Here's how the part is built. I have some questions about the finished solid (model axes, mm). Coordinates: 2 decimals unless noted, no trailing zeros. Write each loop counter-clockwise with the first axis right and the second up, starting at its lowest first coordinate (ties: lowest second). Pieces come first, ordered by that corner, then holes. Notation, with made-up numbers: M -28.5,75.25 L 0.5,75.25 A14 ccw 0.5,99.25 Z; hole C 74,44 d4. An arc over 180 degrees is marked long. Use one line per item in the form item = value. Start each with the question number.
1. Thinking about a two-plate mould opening in Y: for faces 1 (the face through (-2.17, -9.76, 0.49)), 2 (the face through (3.887, -1.591, -4.916)), which applies, released by +Y, released by -Y, zero draft, split by the parting line, or undercut?
2. Please list where these lines run through material, in increasing order: line 1 along Y through (x, z) = (0, -8); line 2 along X through (y, z) = (-6.75, -3); line 3 along Z through (x, y) = (3.5, -8.5). Write a range as [from, to].
3. I want a section at A-A, the plane x = 0. List the corners of the cut face in (y, z) for me.
4. I want a section at C-C, the plane x = 7.75. List the corners of the cut face in (y, z) for me.
5. I want a section at D-D, the plane z = 0.5. Count the separate pieces of the cut face and the enclosed holes in it, plus the area to 3 significant figures.
6. I'm going to push flat-ended pins straight in: pin 1 Ø0.5 at (x, z) = (-7.5, -4) entering from +Y; pin 2 Ø1.3 at (y, z) = (7, -2.5) entering from -X; pin 3 Ø0.5 at (x, z) = (2.5, -2.5) entering from +Y. Where does each tip first touch, or does it pass through?
from build123d import *

# Parameters (mm, degrees)
SKETCH1_R           = 10
BOSS_EXTRUDE1_DEPTH = 1
SKETCH2_R           = 9
BOSS_EXTRUDE2_DEPTH = 11
SKETCH3_R           = 1
CUT_EXTRUDE2_DEPTH  = 19.547236991


with BuildPart() as part:
    # Sketch1 → Boss-Extrude1 (new body)
    with BuildSketch(Plane.XY):
        Circle(SKETCH1_R)
    extrude(amount=BOSS_EXTRUDE1_DEPTH)

    # Sketch2 → Boss-Extrude2 (add)
    with BuildSketch(Plane(origin=(0, 0, 0), x_dir=(-1, 0, 0), z_dir=(0, 0, -1))):
        Circle(SKETCH2_R)
    extrude(amount=BOSS_EXTRUDE2_DEPTH)

    # Sketch3 → Cut-Extrude2 (cut, through all)
    with BuildSketch(Plane.XY.offset(1)):
        Circle(SKETCH3_R)
        with BuildLine():
            ThreePointArc((-1.754992877, 0.4), (-1.272792206, 1.272792206), (-0.4, 1.754992877))
            Line((-0.4, 1.754992877), (-0.4, 3.376388603))
            ThreePointArc((-0.4, 3.376388603), (-2.404163056, 2.404163056), (-3.376388603, 0.4))
            Line((-3.376388603, 0.4), (-1.754992877, 0.4))
        make_face()
        with BuildLine():
            Line((0.4, 3.376388603), (0.4, 1.754992877))
            ThreePointArc((0.4, 1.754992877), (1.272792206, 1.272792206), (1.754992877, 0.4))
            Line((1.754992877, 0.4), (3.376388603, 0.4))
            ThreePointArc((3.376388603, 0.4), (2.404163056, 2.404163056), (0.4, 3.376388603))
        make_face()
        with BuildLine():
            Line((3.376388603, -0.4), (1.754992877, -0.4))
            ThreePointArc((1.754992877, -0.4), (1.272792206, -1.272792206), (0.4, -1.754992877))
            Line((0.4, -1.754992877), (0.4, -3.376388603))
            ThreePointArc((0.4, -3.376388603), (2.404163056, -2.404163056), (3.376388603, -0.4))
        make_face()
        with BuildLine():
            ThreePointArc((-0.4, -1.754992877), (-1.272792206, -1.272792206), (-1.754992877, -0.4))
            Line((-1.754992877, -0.4), (-3.376388603, -0.4))
            ThreePointArc((-3.376388603, -0.4), (-2.404163056, -2.404163056), (-0.4, -3.376388603))
            Line((-0.4, -3.376388603), (-0.4, -1.754992877))
        make_face()
        with BuildLine():
            ThreePointArc((0.4, 4.180908992), (1.607270416, 3.880294037), (2.673506387, 3.239191812))
            Line((2.673506387, 3.239191812), (3.808611797, 4.374297222))
            ThreePointArc((3.808611797, 4.374297222), (2.219563908, 5.358501289), (0.4, 5.786190457))
            Line((0.4, 5.786190457), (0.4, 4.180908992))
        make_face()
        with BuildLine():
            ThreePointArc((-2.673506387, 3.239191812), (-1.607270416, 3.880294037), (-0.4, 4.180908992))
            Line((-0.4, 4.180908992), (-0.4, 5.786190457))
            ThreePointArc((-0.4, 5.786190457), (-2.219563908, 5.358501289), (-3.808611797, 4.374297222))
            Line((-3.808611797, 4.374297222), (-2.673506387, 3.239191812))
        make_face()
        with BuildLine():
            ThreePointArc((-4.180908992, 0.4), (-3.880294037, 1.607270416), (-3.239191812, 2.673506387))
            Line((-3.239191812, 2.673506387), (-4.374297222, 3.808611797))
            ThreePointArc((-4.374297222, 3.808611797), (-5.358501289, 2.219563908), (-5.786190457, 0.4))
            Line((-5.786190457, 0.4), (-4.180908992, 0.4))
        make_face()
        with BuildLine():
            ThreePointArc((-3.239191812, -2.673506387), (-3.880294037, -1.607270416), (-4.180908992, -0.4))
            Line((-4.180908992, -0.4), (-5.786190457, -0.4))
            ThreePointArc((-5.786190457, -0.4), (-5.358501289, -2.219563908), (-4.374297222, -3.808611797))
            Line((-4.374297222, -3.808611797), (-3.239191812, -2.673506387))
        make_face()
        with BuildLine():
            Line((-0.4, -5.786190457), (-0.4, -4.180908992))
            ThreePointArc((-0.4, -4.180908992), (-1.607270416, -3.880294037), (-2.673506387, -3.239191812))
            Line((-2.673506387, -3.239191812), (-3.808611797, -4.374297222))
            ThreePointArc((-3.808611797, -4.374297222), (-2.219563908, -5.358501289), (-0.4, -5.786190457))
        make_face()
        with BuildLine():
            Line((3.808611797, -4.374297222), (2.673506387, -3.239191812))
            ThreePointArc((2.673506387, -3.239191812), (1.607270416, -3.880294037), (0.4, -4.180908992))
            Line((0.4, -4.180908992), (0.4, -5.786190457))
            ThreePointArc((0.4, -5.786190457), (2.219563908, -5.358501289), (3.808611797, -4.374297222))
        make_face()
        with BuildLine():
            Line((5.786190457, -0.4), (4.180908992, -0.4))
            ThreePointArc((4.180908992, -0.4), (3.880294037, -1.607270416), (3.239191812, -2.673506387))
            Line((3.239191812, -2.673506387), (4.374297222, -3.808611797))
            ThreePointArc((4.374297222, -3.808611797), (5.358501289, -2.219563908), (5.786190457, -0.4))
        make_face()
        with BuildLine():
            Line((4.374297222, 3.808611797), (3.239191812, 2.673506387))
            ThreePointArc((3.239191812, 2.673506387), (3.880294037, 1.607270416), (4.180908992, 0.4))
            Line((4.180908992, 0.4), (5.786190457, 0.4))
            ThreePointArc((5.786190457, 0.4), (5.358501289, 2.219563908), (4.374297222, 3.808611797))
        make_face()
        with BuildLine():
            ThreePointArc((8.190238092, 0.4), (7.575812167, 3.138004145), (6.074215607, 5.508530182))
            Line((6.074215607, 5.508530182), (4.941168592, 4.375483167))
            ThreePointArc((4.941168592, 4.375483167), (6.097604915, 2.525710654), (6.587867637, 0.4))
            Line((6.587867637, 0.4), (8.190238092, 0.4))
        make_face()
        with BuildLine():
            ThreePointArc((5.508530182, 6.074215607), (3.138004145, 7.575812167), (0.4, 8.190238092))
            Line((0.4, 8.190238092), (0.4, 6.587867637))
            ThreePointArc((0.4, 6.587867637), (2.525710654, 6.097604915), (4.375483167, 4.941168592))
            Line((4.375483167, 4.941168592), (5.508530182, 6.074215607))
        make_face()
        with BuildLine():
            Line((-0.4, 6.587867637), (-0.4, 8.190238092))
            ThreePointArc((-0.4, 8.190238092), (-3.138004145, 7.575812167), (-5.508530182, 6.074215607))
            Line((-5.508530182, 6.074215607), (-4.375483167, 4.941168592))
            ThreePointArc((-4.375483167, 4.941168592), (-2.525710654, 6.097604915), (-0.4, 6.587867637))
        make_face()
        with BuildLine():
            Line((-4.941168592, 4.375483167), (-6.074215607, 5.508530182))
            ThreePointArc((-6.074215607, 5.508530182), (-7.575812167, 3.138004145), (-8.190238092, 0.4))
            Line((-8.190238092, 0.4), (-6.587867637, 0.4))
            ThreePointArc((-6.587867637, 0.4), (-6.097604915, 2.525710654), (-4.941168592, 4.375483167))
        make_face()
        with BuildLine():
            Line((-6.587867637, -0.4), (-8.190238092, -0.4))
            ThreePointArc((-8.190238092, -0.4), (-7.575812167, -3.138004145), (-6.074215607, -5.508530182))
            Line((-6.074215607, -5.508530182), (-4.941168592, -4.375483167))
            ThreePointArc((-4.941168592, -4.375483167), (-6.097604915, -2.525710654), (-6.587867637, -0.4))
        make_face()
        with BuildLine():
            Line((-4.375483167, -4.941168592), (-5.508530182, -6.074215607))
            ThreePointArc((-5.508530182, -6.074215607), (-3.138004145, -7.575812167), (-0.4, -8.190238092))
            Line((-0.4, -8.190238092), (-0.4, -6.587867637))
            ThreePointArc((-0.4, -6.587867637), (-2.525710654, -6.097604915), (-4.375483167, -4.941168592))
        make_face()
        with BuildLine():
            ThreePointArc((0.4, -8.190238092), (3.138004145, -7.575812167), (5.508530182, -6.074215607))
            Line((5.508530182, -6.074215607), (4.375483167, -4.941168592))
            ThreePointArc((4.375483167, -4.941168592), (2.525710654, -6.097604915), (0.4, -6.587867637))
            Line((0.4, -6.587867637), (0.4, -8.190238092))
        make_face()
        with BuildLine():
            ThreePointArc((6.074215607, -5.508530182), (7.575812167, -3.138004145), (8.190238092, -0.4))
            Line((8.190238092, -0.4), (6.587867637, -0.4))
            ThreePointArc((6.587867637, -0.4), (6.097604915, -2.525710654), (4.941168592, -4.375483167))
            Line((4.941168592, -4.375483167), (6.074215607, -5.508530182))
        make_face()
    extrude(amount=-CUT_EXTRUDE2_DEPTH, mode=Mode.SUBTRACT)


solid = part.part
Answer list:
q1.face_1 = split by the parting line
q1.face_2 = undercut
q2.line_1 = [-9, -1], [1, 9]
q2.line_2 = [-5.95, -4.66], [-0.4, 0.4], [4.66, 5.95]
q2.line_3 = [0, 1]
q3.outline = M -10,0 L -9,0 L -9,-11 L -1,-11 L -1,1 L -10,1 Z; M 1,-11 L 9,-11 L 9,0 L 10,0 L 10,1 L 1,1 Z
q4.outline = M -6.32,0 L -4.58,0 L -4.58,-11 L -2.68,-11 L -2.68,1 L -6.32,1 Z; M -0.4,-11 L 0.4,-11 L 0.4,1 L -0.4,1 Z; M 2.68,-11 L 4.58,-11 L 4.58,0 L 6.32,0 L 6.32,1 L 2.68,1 Z
q5.separate_pieces = 1
q5.enclosed_holes = 21
q5.area = 186 mm²
q6.pin_1 = 5.33
q6.pin_2 = -6.38
q6.pin_3 = 8.71
